Check sheet for the modelled part. Datum: model origin and axes. Units: mm. A direction names the side the tool comes from. Round coordinates to 2 decimals unless told otherwise and drop trailing zeros. Loops run counter-clockwise (first coordinate to the right, second up) from the corner with the lowest first, then second, coordinate; pieces in that order, holes last. Notation, with made-up numbers: M 29.25,23 L 69.25,23 A26 ccw 69.25,53 Z; hole C -33.5,3 d2. An arc over 180 degrees is marked long. Write item = value, one per line. Start each with the question number.
(1) Scan lines: L1, parallel to X at y = 0, z = 0.05; L2, parallel to Y at x = 32.5, z = 0; L3, parallel to Z at x = 33, y = 1.3. Record each from-to range of solid material in increasing order. Write a range as from..to.
(2) Cross-section at B-B on x = 27.5. Record the boundary of the cut face in (y, z).
(3) Set-up check for faces 1 (the face through (24.25, 0, 1)), 2 (the face through (32.5, 1.3, -0.1)), 3 (the face through (15.28, -1.5, -0.07)): record each of +Z, -Z, +X, -X, +Y, -Y from which the full face is reachable in a straight line by a thin tool's end or side.
(4) Go/stop test with flat-tipped pins: P1, Ø1, axis at y = -0.5, z = -1, coming from the +X side; P2, Ø0.9, axis at x = 33, y = -0.5, coming from the -Z side; P3, Ø1.5, axis at x = 30.5, y = 0, coming from the +Z side. Record where each tip stops, or that it passes through.
(5) Cross-section at A-A on y = 0. State how many separate pieces and enclosed holes the cut face has, plus the area to 3 significant figures.
(6) Cross-section at C-C on z = 0.95. Record the boundary of the cut face in (x, y).
(7) Cross-section at D-D on x = 4.5. Record the boundary of the cut face in (y, z), plus the area to 3 significant figures.
Autodesk Inventor part; units mm, degrees
ref_plane "Work Plane1" through (0, 0, -1.5) normal (0, 0, 1) x (1, 0, 0)
ref_plane "Work Plane2" through (0, 0, 0) normal (0, 0.7071, 0.7071) x (1, 0, 0)
ref_plane "YZ Plane" through (0, 0, 0) normal (1, 0, 0) x (0, 1, 0)
sketch "Sketch1" plane through (0, 0, 0) normal (1, 0, 0) x (0, 1, 0)
  circle A0 centre (0, 0) radius 1.5
  dimension "d0" = 3
extrude "Extrusion1" add sketch "Sketch1" along normal blind 71
ref_plane "Work Plane1" through (0, 0, -1.5) normal (0, 0, 1) x (1, 0, 0)
sketch "Sketch3" plane through (0, 0, -1.5) normal (0, 0, 1) x (1, 0, 0)
  line L0 (-14.2, 0) -> (85.2, 0) construction
  line L1 (0, -1.5) -> (0, 1.5) construction
  point P0 (0, 0)
  point P1 (27.5, 0)
  dimension "d16" = 27.5
hole "Hole1" at (27.5, 0, -1.5) direction (0, 0, 1) diameter 2 end through all
pattern_linear "Rectangular Pattern1" count 5 spacing 2.5 along (1, 0, 0) of "Hole1"
sketch "Sketch2" plane through (0, 0, 0) normal (0, 1, 0) x (-1, 0, 0)
  line L0 (-71, 1.5) -> (-71, -1.5) construction
  line L1 (0, 1.5) -> (0, -1.5) construction
  line L2 (-24.25, 1.5) -> (-40.75, 1.5)
  line L3 (-40.75, 1.5) -> (-40.75, 0.6)
  line L4 (-40.25, 0.1) -> (-24.75, 0.1)
  line L5 (-24.25, 0.6) -> (-24.25, 1.5)
  line L6 (-24.25, -1.5) -> (-40.75, -1.5)
  line L7 (-40.75, -1.5) -> (-40.75, -0.6)
  line L8 (-40.25, -0.1) -> (-24.75, -0.1)
  line L9 (-24.25, -0.6) -> (-24.25, -1.5)
  line L10 (0, 1.5) -> (-71, 1.5) construction
  line L11 (0, -1.5) -> (-71, -1.5) construction
  line L12 (13.2, 0) -> (-79.2, 0) construction
  arc A0 (-24.75, 0.1) -> (-24.25, 0.6) centre (-24.75, 0.6) ccw
  arc A1 (-40.75, 0.6) -> (-40.25, 0.1) centre (-40.25, 0.6) ccw
  arc A2 (-24.25, -0.6) -> (-24.75, -0.1) centre (-24.75, -0.6) ccw
  arc A3 (-40.25, -0.1) -> (-40.75, -0.6) centre (-40.25, -0.6) ccw
  point P0 (0, 0)
  dimension "d3" = 0.5
  dimension "d4" = 0.2
  dimension "d20" = 16.5
  dimension "d21" = 24.25
extrude "Extrusion2" cut sketch "Sketch2" along normal through all both and the other way through all
ref_plane "Work Plane2" through (0, 0, 0) normal (0, 0.7071, 0.7071) x (1, 0, 0)
sketch "Sketch4" plane through (0, 0, 0) normal (0, 0.7071, 0.7071) x (1, 0, 0)
  line L0 (26.9374, -0.3516) -> (28.0626, -0.3516)
  line L1 (28.0626, -0.3516) -> (28.0626, 0.3516)
  line L2 (28.0626, 0.3516) -> (26.9374, 0.3516)
  line L3 (26.9374, 0.3516) -> (26.9374, -0.3516)
  line L4 (26.9374, -0.3516) -> (28.0626, 0.3516) construction
  line L5 (28.0626, -0.3516) -> (26.9374, 0.3516) construction
  line L6 (26.7934, -0.5175) -> (28.2066, -0.5175)
  line L7 (28.2066, -0.5175) -> (28.2066, 0.5175)
  line L8 (28.2066, 0.5175) -> (26.7934, 0.5175)
  line L9 (26.7934, 0.5175) -> (26.7934, -0.5175)
  line L10 (26.7934, -0.5175) -> (28.2066, 0.5175) construction
  line L11 (28.2066, -0.5175) -> (26.7934, 0.5175) construction
  line L12 (27.1467, -0.2588) -> (27.8533, -0.2588)
  line L13 (27.8533, -0.2588) -> (27.8533, 0.2587)
  line L14 (27.8533, 0.2587) -> (27.1467, 0.2587)
  line L15 (27.1467, 0.2587) -> (27.1467, -0.2588)
  line L16 (27.1467, -0.2588) -> (27.8533, 0.2587) construction
  line L17 (27.8533, -0.2588) -> (27.1467, 0.2587) construction
  line L18 (-5.7, 0) -> (34.2, 0) construction
  ellipse E0 centre (27.5, -0.0707) end of major axis (28.5, -0.0707) minor radius 0.7071 construction
  ellipse E1 centre (27.5, 0.0707) end of major axis (28.5, 0.0707) minor radius 0.7071 construction
  line L19 (27.5, -0.0707) -> (27.5, 0.0707) construction
  point P0 (0, 0)
  point P1 (27.5, 0)
  dimension "d23" = 0.7032
  dimension "d24" = 1.1251
  dimension "d25" = 1.4131
  dimension "d26" = 1.035
  dimension "d27" = 0.5175
  dimension "d28" = 0.7066
sketch "Sketch5" plane through (71, 0, 0) normal (1, 0, 0) x (0, 0, -1)
  circle A0 centre (0, 0) radius 1.5
extrude "Extrusion3" cut sketch "Sketch5" against normal blind 31
equation "\"d9\" = DiameterHole"
equation "\"d19\" = DistanceHoleHole"
equation "\"d4\" = Thickness"
equation "\"DistanceHoleHole\" = 2.5"
equation "\"DiameterHole\" = 2"
equation "\"DistanceHoleEnd\" = 27.5"
equation "\"Thickness\" = 0.2"
properties part number "5_multi_beetle_holder"
Result:
q1.L1 = 0..26.5, 28.5..29, 31..31.5, 33.5..34, 36..36.5, 38.5..40
q1.L2 = -1.5..-1, 1..1.5
q1.L3 = -0.1..0.1
q2.outline = M -1.5,-0.1 L -1,-0.1 L -1,0.1 L -1.5,0.1 A1.5 ccw Z; M 1,-0.1 L 1.5,-0.1 A1.5 ccw 1.5,0.1 L 1,0.1 Z
q3.face_1 = +Z, +X, +Y, -Y
q3.face_2 = -Z, +X, +Y, -Y
q3.face_3 = +X, -X
q4.P1 = 24.26
q4.P2 = -0.1
q4.P3 = 0.1
q5.separate_pieces = 6
q5.enclosed_holes = 0
q5.area = 74.0 mm^2
q6.outline = M 0,-1.16 L 24.25,-1.16 L 24.25,1.16 L 0,1.16 Z
q7.outline = C 0,0 d3
q7.area = 7.07 mm^2
